from build123d import *

# Parameters (mm, degrees)
SKETCH1_W           = 308
SKETCH1_H           = 108
BOSS_EXTRUDE1_DEPTH = 6
CUT_EXTRUDE1_DEPTH  = 10
SKETCH3_R           = 3.4
CUT_EXTRUDE2_DEPTH  = 7


with BuildPart() as part:
    # Sketch1 → Boss-Extrude1 (new body)
    with BuildSketch(Plane(origin=(0, 0, 0), x_dir=(1, 0, 0), z_dir=(0, 1, 0))):
        Rectangle(SKETCH1_W, SKETCH1_H)
    extrude(amount=BOSS_EXTRUDE1_DEPTH)

    # Sketch2 → Cut-Extrude1 (cut)
    with BuildSketch(Plane.XZ):
        with BuildLine():
            Line((-25, -20), (25, -20))
            ThreePointArc((25, -20), (32.071067812, -17.071067812), (35, -10))
            Line((35, -10), (35, 10))
            ThreePointArc((35, 10), (32.071067812, 17.071067812), (25, 20))
            Line((25, 20), (-25, 20))
            ThreePointArc((-25, 20), (-32.071067812, 17.071067812), (-35, 10))
            Line((-35, 10), (-35, -10))
            ThreePointArc((-35, -10), (-32.071067812, -17.071067812), (-25, -20))
        make_face()
    extrude(amount=-CUT_EXTRUDE1_DEPTH, mode=Mode.SUBTRACT)

    # Sketch3 → Cut-Extrude2 (cut, through all)
    with BuildSketch(Plane(origin=(0, 0, 0), x_dir=(-1, 0, 0), z_dir=(0, -1, 0))):
        with Locations((41, -21)):
            Circle(SKETCH3_R)
        with Locations((-41, -21)):
            Circle(SKETCH3_R)
        with Locations((-41, 21)):
            Circle(SKETCH3_R)
        with Locations((41, 21)):
            Circle(SKETCH3_R)
    extrude(amount=-CUT_EXTRUDE2_DEPTH, mode=Mode.SUBTRACT)


solid = part.part
Design review of the part built by this model. Coordinates are the model's own, in mm. A direction names the side the tool comes from. Coordinates: 2 decimals unless noted, no trailing zeros. Loops run counter-clockwise (first coordinate to the right, second up) from the corner with the lowest first, then second, coordinate; pieces in that order, holes last.
Item 1: Add section A-A (x = -4). Write out the cut boundary in (y, z).
Completed:
outline: (0, -54) - (6, -54) - (6, -20) - (0, -20) - close; (0, 20) - (6, 20) - (6, 54) - (0, 54) - close
Item 2: Draft analysis for pull direction Z (two halves, no side actions). For faces 3 (the flat face through (-154, 3, 1)), 4 (the cylindrical face through (-44.14, 2.96, -19.7)), 5 (the flat face through (-2, 3, -54)), state which applies: pulls with the +Z half, pulls with the -Z half, needs draft (parallel to the pull), parting line crosses it, or undercut.
Completed:
face 3: needs draft
face 4: undercut
face 5: pulls with the -Z half
Item 3: For faces 1 (the flat face through (0, 3, 20)), 2 (the flat face through (154, 3, 1)), list the 3-axis set-ups (+Z, -Z, +X, -X, +Y, -Y) from which the entire face can be reached by the end or side of a thin tool; tool diameter is ignored.
Completed:
face 1: +Y, -Y
face 2: +Z, -Z, +X, +Y, -Y
Item 4: Clearance check with a flat-ended pin moving along its axis: pin 1 (4 mm diameter, centred on x = 41, z = -21, fed in from -Y). State where the tip first meets the part, or that it passes through.
Completed:
pin 1: passes through
Item 5: Add section B-B (y = 4.9). Write out the cut boundary in (x, z), and give its area (3 significant figures).
Completed:
outline: (-154, -54) - (154, -54) - (154, 54) - (-154, 54) - close; hole circle Ø6.8 at (-41, -21); hole circle Ø6.8 at (-41, 21); hole (-35, -10) arc R10 ccw to (-25, -20) - (25, -20) arc R10 ccw to (35, -10) - (35, 10) arc R10 ccw to (25, 20) - (-25, 20) arc R10 ccw to (-35, 10) - close; hole circle Ø6.8 at (41, -21); hole circle Ø6.8 at (41, 21)
area: 30,400 mm2
Item 6: Add section C-C (x = -41). Write out the cut boundary in (y, z).
Completed:
outline: (0, -54) - (6, -54) - (6, -24.4) - (0, -24.4) - close; (0, -17.6) - (6, -17.6) - (6, 17.6) - (0, 17.6) - close; (0, 24.4) - (6, 24.4) - (6, 54) - (0, 54) - close
Item 7: Wall thickness on L1, parallel to Z at x = -41, y = 1.55; L2, parallel to X at y = 2.7, z = 21; L3, parallel to Z at x = -4, y = 0.3: over which ranges is each line inside the solid? List them lowest first.
Completed:
L1: z = -54 to -24.4, -17.6 to 17.6, 24.4 to 54
L2: x = -154 to -44.4, -37.6 to 37.6, 44.4 to 154
L3: z = -54 to -20, 20 to 54
Item 8: Add section D-D (z = 0.5). Write out the cut boundary in (x, y).
Completed:
outline: (-154, 0) - (-35, 0) - (-35, 6) - (-154, 6) - close; (35, 0) - (154, 0) - (154, 6) - (35, 6) - close
